from build123d import *

# Parameters (mm, degrees)
F0_W           = 172
F0_H           = 60.5
F4_DEPTH       = 5
F6_SIZE2       = 4
F6_SIZE        = 3
F9_DEPTH       = 5
F10_SIZE       = 4.99999
F11_SIZE2      = 0.99999
F11_SIZE       = 4.99999
F12_SIZE       = 1
F14_W          = 132
F14_H          = 20.5
F15_DEPTH      = 12.5
F17_DEPTH      = 25
F17_DEPTH_BACK = 25


# Not quite as in the source:
# - a fillet or chamfer is up to 0.001 mm smaller than in the source, because OpenCascade refuses the exact size


with BuildPart() as f4:
    # F0 (on Top) → F4 (new body)
    with BuildSketch(Plane.XY):
        Rectangle(F0_W, F0_H)
    extrude(amount=-F4_DEPTH)

    # F3 (on Top) → F5 section 0
    with BuildSketch(Plane.XY):
        Polygon((-86, 0), (-86, -30.25), (-55.75, -30.25), (-55.75, -20.25), (-76, -20.25), (-76, 0), align=None)
    # F2 (on offset) → F5 section 1
    with BuildSketch(Plane.XY.offset(15)):
        Polygon((-76, -20.25), (-76, 0), (-81, 0), (-81, -25.25), (-66, -25.25), (-66, -20.25), align=None)
    loft()

    # F6
    f6_edges = [f4.edges().sort_by_distance(p)[0] for p in [
        (-76, -10.125, 15),
        (-71, -20.25, 15),
    ]]
    chamfer(f6_edges, length=F6_SIZE, length2=F6_SIZE2)

    # F7: F4 across plane


with BuildPart() as f4_1:
    add(f4.part)
    add(f4.part.mirror(Plane.YZ))

    # F8 (on face) → F9 (join)
    with BuildSketch(Plane.XY):
        Polygon((13.8189587742, -20.25), (0, -20.25), (-13.8189587742, -20.25), (-13.8189587742, -30.1344580948), (0, -30.1344580948), (13.8189587742, -30.1344580948), align=None)
    extrude(amount=F9_DEPTH)

    # F10 (size 5 in the source; OpenCascade refuses exactly that, so slightly less here)
    f10_edges = [f4_1.edges().sort_by_distance(p)[0] for p in [
        (13.818959, -25.192229, 5),
        (0, -30.134458, 5),
        (-13.818959, -25.192229, 5),
    ]]
    chamfer(f10_edges, length=F10_SIZE)

    # F11 (size 5 and 1 in the source; OpenCascade refuses exactly that, so slightly less here)
    f11_edges = [f4_1.edges().sort_by_distance(p)[0] for p in [
        (0, -20.25, 5),
    ]]
    f11_side = f4_1.faces().sort_by_distance((0, -20.25, 2.315943))[0]
    chamfer(f11_edges, length=F11_SIZE, length2=F11_SIZE2, reference=f11_side)

    # F12
    f12_edges = [f4_1.edges().sort_by_distance(p)[0] for p in [
        (0, -21.24999, 5),
    ]]
    chamfer(f12_edges, length=F12_SIZE)

    # F13: F4 across plane


with BuildPart() as f4_2:
    add(f4_1.part)
    add(f4_1.part.mirror(Plane.XZ))

    # F14 (on Top) → F15 (cut, symmetric)
    with BuildSketch(Plane.XY):
        Rectangle(F14_W, F14_H)
    extrude(amount=F15_DEPTH, both=True, mode=Mode.SUBTRACT)


with BuildPart() as f17:
    # F16 (on Top) → F17 (new body, two sides)
    with BuildSketch(Plane.XY) as f17_sk:
        Polygon((23.7979591321, 44.0479591321), (0, 20.25), (18.644013716, 1.605986284), (18.644013716, -1.605986284), (0, -20.25), (26.894013716, -47.144013716), (91.0670285058, -47.144013716), (91.0670285058, 44.0479591321), align=None)
    extrude(amount=F17_DEPTH)
    extrude(f17_sk.sketch, amount=-F17_DEPTH_BACK)


with BuildPart() as f4_3:
    add(f4_2.part)

    # F18: cut F17
    add(f17.part, mode=Mode.SUBTRACT)


solid = f4_3.part
Input: part model. Units: mm. Frame: model coordinates. A direction names the side the tool comes from. Round coordinates to 2 decimals unless told otherwise and drop trailing zeros. Order: outer loops, then holes, each group sorted by start corner. A loop starts at its lowest first (then second) coordinate and runs counter-clockwise, first axis right, second up. Notation, with made-up numbers: (75, -34) - (112, -34) arc R19 ccw to (112, -25) - close; hole circle Ø4 at (22, 73). An arc over 180 degrees is marked (long way). Use a Markdown table: item, result.
1. Section D-D on x = -35.5. Return the cut outline in (y, z).
Evaluation:
| item | result |
|---|---|
| outline | (-30.25, -5) - (-10.25, -5) - (-10.25, 0) - (-30.25, 0) - close; (10.25, -5) - (30.25, -5) - (30.25, 0) - (10.25, 0) - close |
2. Mould query, pull axis Y, two halves, no side actions, for faces 1 (the face through (-2, -24, 5)), 2 (the face through (-2.133, 27.599, 2.535)), 3 (the face through (-29, -10.25, -2)). Classes: +Y half, -Y half, draft (parallel to the pull), parting line (faces both ways), or undercut.
Evaluation:
| item | result |
|---|---|
| face 1 | draft |
| face 2 | +Y half |
| face 3 | undercut |
3. First-contact query: pin 1 (1.4 mm diameter, centred on x = -3, y = 23.5, fed in from +Z); pin 2 (1.5 mm diameter, centred on y = 7.5, z = 3, fed in from -X); pin 3 (18 mm diameter, centred on x = -47, y = -9.5, fed in from +Z). Flat tips, straight axial feed; report the tip coordinate or a pass-through.
Evaluation:
| item | result |
|---|---|
| pin 1 | z = 5 |
| pin 2 | x = -85.25 |
| pin 3 | z = 0 |
4. Material intervals for probe 1 along Y at (x, z) = (-30.5, -2.5); probe 2 along Z at (x, y) = (-17, 16); probe 3 along X at (y, z) = (-7, -3), sorted ascending.
Evaluation:
| item | result |
|---|---|
| probe 1 | -30.25 to -10.25, 10.25 to 30.25 |
| probe 2 | -5 to 0 |
| probe 3 | -86 to -66 |
5. Access query for faces 4 (the face through (-29, 10.25, -2)), 5 (the face through (-11.84, 24.02, 1.98)), 6 (the face through (-76, 0, 6)). Directions: +Z, -Z, +X, -X, +Y, -Y. A direction counts if a zero-diameter tool reaches every point of the face in a straight line with its end or side. Return the directions, or none.
Evaluation:
| item | result |
|---|---|
| face 4 | +Z, -Z, +X |
| face 5 | +Z, +Y, -Y |
| face 6 | +Z, +X |
6. Section B-B on y = -18. Return the cut outline in (x, z).
Evaluation:
| item | result |
|---|---|
| outline | (-86, -5) - (2.25, -5) - (2.25, 0) - (-76, 0) - (-76, 11) - (-79, 15) - (-81, 15) - (-86, 0) - close |
7. Section C-C on z = -2.25. Return the cut outline in (x, y), then the cut area to 3 significant figures.
Evaluation:
| item | result |
|---|---|
| outline | (-86, -30.25) - (10, -30.25) - (0, -20.25) - (10, -10.25) - (-66, -10.25) - (-66, 10.25) - (10, 10.25) - (0, 20.25) - (10, 30.25) - (-86, 30.25) - close |
| area | 4,050 mm^2 |
